The listing builds one solid part. Answer for the finished solid, in the listing's coordinates (mm). Give positions to 0.01 mm unless a question says otherwise; leave off trailing zeros. Write each loop counter-clockwise with the first axis right and the second up, starting at its lowest first coordinate (ties: lowest second). Pieces come first, ordered by that corner, then holes. Notation, with made-up numbers: M 63,-10 L 84,-10 A26 cw 84,25 Z; hole C 10.25,14.25 d2. An arc over 180 degrees is marked long. Return JSON: item names as keys, results as strings.
from build123d import *

# Parameters (mm, degrees)
ESQUISSE1_W             = 25.4
ESQUISSE1_H             = 25.4
BOSS_EXTRU_1_DEPTH      = 14.81582
BOSS_EXTRU_1_TAPER      = 40.5
ESQUISSE2_R             = 1.666875
ENL_V_MAT_EXTRU_1_DEPTH = 12.7


with BuildPart() as part:
    # Esquisse1 → Boss.-Extru.1 (new body)
    with BuildSketch(Plane.XY):
        Rectangle(ESQUISSE1_W, ESQUISSE1_H)
    extrude(amount=BOSS_EXTRU_1_DEPTH, taper=BOSS_EXTRU_1_TAPER)

    # Esquisse2 → Enlèv. mat.-Extru.1 (cut)
    with BuildSketch(Plane(origin=(0, -12.7, 0), x_dir=(1, 0, 0), z_dir=(0, 1, 0))):
        with Locations(Location((0, -7.40791, 0), (0, 0, 90))):
            Circle(ESQUISSE2_R)
    extrude(amount=ENL_V_MAT_EXTRU_1_DEPTH, mode=Mode.SUBTRACT)


solid = part.part
Item 1: Determine the mould class of faces 1 (the flat face through (7.868, 0.178, 5.658)), 2 (the flat face through (-7.868, -0.178, 5.658)), 3 (the cylindrical face through (0.64, -3.09, 5.87)) for opening direction X: +X half, -X half, draft (parallel to the pull), parting line (faces both ways), or undercut.
Geometry results:
{"face 1": "+X half", "face 2": "-X half", "face 3": "undercut"}
Item 2: Given pin 1 Ø4 at (x, z) = (-4, 11) entering from -Y; pin 2 Ø1.5 at (x, z) = (-5.5, 6.5) entering from +Y; pin 3 Ø1.5 at (x, z) = (1, 2) entering from -Y, each flat-ended and moving along its own axis, determine where each tip first touches the part or whether it passes through.
Geometry results:
{"pin 1": "stops at y = -5.01", "pin 2": "stops at y = 7.79", "pin 3": "stops at y = -11.63"}
Item 3: A cutting plane is placed at A-A, the plane y = -1. Write down the section's boundary in (x, z).
Geometry results:
{"outline": "M -12.7,0 L 12.7,0 L 1,13.7 L -1,13.7 Z; hole C 0,7.41 d3.33"}
Item 4: A cutting plane is placed at C-C, the plane z = 2.5. Write down the section's boundary in (x, y), plus the area to 3 significant figures.
Geometry results:
{"outline": "M -10.56,-10.56 L 10.56,-10.56 L 10.56,10.56 L -10.56,10.56 Z", "area": "446 mm2"}
Item 5: Find the intervals of material crossed by line 1 (X direction, y = -5, z = 6.25); line 2 (Z direction, x = -9.5, y = 4.5); line 3 (X direction, y = 3, z = 11), in increasing order.
Geometry results:
{"line 1": "x = -7.36 to -1.2, 1.2 to 7.36", "line 2": "z = 0 to 3.75", "line 3": "x = -3.31 to 3.31"}
Item 6: A cutting plane is placed at B-B, the plane x = 5.25. Write down the section's boundary in (y, z).
Geometry results:
{"outline": "M -12.7,0 L 12.7,0 L 5.25,8.72 L -5.25,8.72 Z"}
